The model under review builds one solid part; all positions refer to its coordinate system, in mm. A direction names the side the tool comes from. Round coordinates to 2 decimals unless told otherwise and drop trailing zeros. Loops run counter-clockwise (first coordinate to the right, second up) from the corner with the lowest first, then second, coordinate; pieces in that order, holes last. Notation, with made-up numbers: M 78.5,16 L 121.5,16 A30 cw 121.5,46 Z; hole C 55,12 d5. An arc over 180 degrees is marked long. Answer as a JSON object with one key per item and string values. Group by question number.
Item 1: To check wall thickness, follow line 1 (Y direction, x = -57, z = 9.5); line 2 (X direction, y = 184, z = 1); line 3 (X direction, y = 54, z = 6). State the ranges of each line that lie inside material, in increasing order.
Item 2: Consider section D-D (y = 131). Give the boundary of the cut face in (x, z), and give its area (3 significant figures).
Item 3: The part is to be moulded in two halves that separate along X. For faces 3 (the face through (60, 137, 8)), 4 (the face through (55, 135, 9)), 5 (the face through (-1, 92, 0)), 6 (the face through (-60, 135, 8)), say which applies: +X half, -X half, draft (parallel to the pull), parting line (faces both ways), or undercut.
Item 4: Tool access review of faces 1 (the face through (57.535, 153.585, 4.881)), 2 (the face through (-1, 92, 2)): name each direction out of +Z, -Z, +X, -X, +Y, -Y from which nothing blocks a thin tool from reaching the whole face with its end or side.
Item 5: Consider section A-A (y = 155.5). Give the boundary of the cut face in (x, z), and give its area (3 significant figures).
Item 6: Insertion check: P1, Ø6, axis at x = 16.5, y = 55.5, coming from the +Z side; P2, Ø5.5, axis at x = -56.5, z = 9.5, coming from the -Y side; P3, Ø1, axis at x = -49.5, z = 1.5, coming from the +Y side. Each pin has a flat end and moves straight along its axis. Give the tip position at first contact, or say it passes through.
Item 7: Consider section B-B (y = 192.5). Give the boundary of the cut face in (x, z).
Item 8: Consider section C-C (z = 9.5). Give the boundary of the cut face in (x, y).
Autodesk Inventor part; units mm, degrees
ref_plane "工作平面1" through (31, 232, 17) normal (1, 0, 0) x (0, 0, -1)
ref_plane "YZ Plane" through (0, 0, 0) normal (1, 0, 0) x (0, 1, 0)
ref_plane "XZ Plane" through (0, 0, 0) normal (0, 1, 0) x (-1, 0, 0)
sketch "草图1" plane through (0, 0, 0) normal (0, 0, 1) x (1, 0, 0)
  line L0 (-60, 0) -> (60, 0)
  line L1 (-60, 0) -> (-60, 232)
  line L2 (-60, 232) -> (60, 232)
  line L3 (60, 232) -> (60, 0)
  point P0 (0, 0)
  point P1 (0, 0)
  dimension "宽度" = 120
  dimension "长度" = 232
  dimension "d15" = 120
extrude "拉伸1" add sketch "草图1" along normal blind 2
sketch "草图2" plane through (0, 0, 2) normal (0, 0, 1) x (1, 0, 0)
  line L0 (-60, 0) -> (60, 0)
  line L1 (60, 0) -> (60, 232)
  line L2 (60, 232) -> (-60, 232)
  line L3 (-60, 232) -> (-60, 0)
  line L4 (-55, 232) -> (-55, 0)
  line L5 (0, 0) -> (0, 232) construction
  line L6 (55, 0) -> (55, 232)
  dimension "侧厚" = 5
extrude "拉伸2" add sketch "草图2" along normal blind 15 contours L3 L2 L4 L0 | L6 L2 L1 L0
sketch "草图3" plane through (60, 0, 0) normal (1, 0, 0) x (0, 0, -1)
  line L0 (0, 0) -> (0, 232)
  line L1 (0, 232) -> (-17, 232)
  line L2 (-17, 0) -> (-17, 232)
  line L3 (0, 0) -> (-17, 0)
  circle A0 centre (-9.5, 222) radius 5
  circle A1 centre (-9.5, 155.5) radius 5
  line L4 (-9.5, 222) -> (-9.5, 155.5) construction
  point P0 (0, 0)
  dimension "d16" = 10
  dimension "后孔位置" = 10
  dimension "上沿" = 7.5
  dimension "d29" = 10
  dimension "d30" = 66.5
extrude "拉伸3" cut sketch "草图3" against normal through all contours A0
sketch "草图4" plane through (0, 0, 2) normal (0, 0, 1) x (1, 0, 0)
  line L0 (-52, 232) -> (-52, 187)
  line L1 (-52, 187) -> (52, 187)
  line L2 (52, 187) -> (52, 232)
  line L3 (55, 232) -> (-55, 232)
  line L4 (0, 232) -> (0, 179.736464)
  line L5 (-52, 232) -> (52, 232)
  line L6 (55, 232) -> (55, 0)
  point P0 (0, 0)
  dimension "d26" = 45
  dimension "d39" = 3
extrude "拉伸4" cut sketch "草图4" along normal through all both and the other way through all
extrude "拉伸5" cut sketch "草图3" against normal through all contours A1
sketch "草图5" plane through (0, 0, 2) normal (0, 0, 1) x (1, 0, 0)
  line L0 (-55, 0) -> (-55, 232)
  line L1 (-52, 232) -> (-55, 232)
  line L2 (-45, 232) -> (-45, 92)
  line L3 (-25, 232) -> (-25, 92)
  line L4 (-45, 92) -> (-25, 92)
  point P0 (0, 0)
  dimension "d33" = 140
  dimension "d34" = 10
  dimension "d35" = 140
  dimension "d36" = 20
sketch "草图5 outline for 拉伸6" plane through (0, 0, 2) normal (0, 0, 1) x (1, 0, 0)
  line L0 (-45, 232) -> (-25, 232)
  line L1 (-25, 232) -> (-25, 92)
  line L2 (-25, 92) -> (-45, 92)
  line L3 (-45, 92) -> (-45, 232)
extrude "拉伸6" cut sketch "草图5 outline for 拉伸6" along normal through all both and the other way through all
sketch "草图6" plane through (0, 0, 2) normal (0, 0, 1) x (1, 0, 0)
  line L0 (60, 160.5) -> (60, 150.5)
  line L1 (55, 150.5) -> (55, 160.5)
  line L2 (55, 155.5) -> (0, 155.5) construction
  line L3 (0, 145.5) -> (0, 0) construction
  line L4 (55, 155.5) -> (55, 95.5) construction
  line L5 (55, 95.5) -> (0, 95.5) construction
  line L6 (-10, 95.5) -> (10, 95.5)
  line L7 (52, 187) -> (-25, 187)
  line L8 (10, 145.5) -> (10, 177) construction
  line L9 (0, 187) -> (0, 97)
  line L10 (0, 97) -> (20, 97)
  line L11 (20, 97) -> (20, 187)
  dimension "d40" = 60
  dimension "d46" = 90
  dimension "d47" = 20
  dimension "d48" = 10
extrude "拉伸7" cut sketch "草图6" against normal through all
sketch "草图7" plane through (0, 0, 2) normal (0, 0, 1) x (1, 0, 0)
  line L0 (60, 227) -> (60, 217)
  line L1 (55, 217) -> (55, 227)
  line L2 (-60, 232) -> (-60, 0)
  line L3 (60, 0) -> (60, 232)
  line L4 (-60, 0) -> (60, 0)
  line L5 (55, 222) -> (60, 222) construction
  circle A0 centre (0, 10) radius 2.5
  point P0 (0, 0)
  dimension "d49" = 5
  dimension "d50" = 212
extrude "拉伸8" cut sketch "草图7" against normal through all
sketch "草图8" plane through (0, 0, 2) normal (0, 0, 1) x (1, 0, 0)
  circle A0 centre (0, 10) radius 2.5
  line L0 (20, 187) -> (20, 97)
  line L1 (20, 97) -> (0, 97)
  line L2 (0, 97) -> (0, 187)
  line L3 (0, 187) -> (-25, 187)
  line L4 (-25, 187) -> (-25, 92)
  line L5 (-25, 92) -> (-45, 92)
  line L6 (-45, 92) -> (-45, 187)
  line L7 (-45, 187) -> (-52, 187)
  line L8 (-52, 187) -> (-52, 232)
  line L9 (-52, 232) -> (-55, 232)
  line L10 (-55, 232) -> (-55, 0)
  line L11 (-55, 0) -> (55, 0)
  line L12 (55, 0) -> (55, 232)
  line L13 (55, 232) -> (52, 232)
  line L14 (52, 232) -> (52, 187)
  line L15 (52, 187) -> (20, 187)
  line L16 (-60, 0) -> (-55, 0)
  line L17 (-55, 0) -> (-55, 232)
  line L18 (-55, 232) -> (-60, 232)
  line L19 (-60, 232) -> (-60, 0)
  line L20 (60, 0) -> (60, 232)
  line L21 (60, 232) -> (55, 232)
  line L22 (55, 232) -> (55, 0)
  line L23 (55, 0) -> (60, 0)
  line L24 (-15, 0) -> (-55, 40)
  line L25 (15, 0) -> (55, 40)
  line L26 (0, 0) -> (0, 39.183664) construction
  line L27 (-60, 232) -> (-60, 0)
  line L28 (-55, 40) -> (-60, 40)
  line L29 (-60, 40) -> (-60, 0)
  line L30 (-60, 0) -> (-15, 0)
  line L31 (15, 0) -> (60, 0)
  line L32 (55, 40) -> (60, 40)
  line L33 (60, 0) -> (60, 40)
  dimension "d53" = 30
  dimension "d55" = 40
extrude "拉伸9" cut sketch "草图8" along normal through all both and the other way through all contours L32 L20 L23 L12 | L12 L11 L25 | L11 L10 L24 | L16 L19 L28 L10
ref_plane "工作平面1" through (31, 232, 17) normal (1, 0, 0) x (0, 0, -1)
sketch "草图9" plane through (31, 232, 17) normal (1, 0, 0) x (0, 0, -1)
  line L0 (17, -192) -> (17, 0)
  line L1 (17, -56.209089) -> (-323, -175.94833)
  line L2 (-322.950917, -180.94833) -> (17, -61.209089)
  line L3 (17, -56.209089) -> (17, -61.209089)
  line L4 (-322.950917, -180.94833) -> (-323, -175.94833)
  point P0 (17, -232)
  dimension "d59" = 340
  dimension "d64" = 5
  dimension "d65" = 5
extrude "拉伸11" [suppressed]
properties part number "底板" material "木材(桦木)"
Geometry results:
{
 "1": {"line 1": "y = 40 to 150.5, 160.5 to 217, 227 to 232", "line 2": "x = -60 to -45, -25 to 0, 20 to 60", "line 3": "x = -60 to -55, 55 to 60"},
 "2": {"outline": "M -60,0 L -45,0 L -45,2 L -55,2 L -55,17 L -60,17 Z; M -25,0 L 0,0 L 0,2 L -25,2 Z; M 20,0 L 60,0 L 60,17 L 55,17 L 55,2 L 20,2 Z", "area": "310 mm^2"},
 "3": {"face 3": "+X half", "face 4": "undercut", "face 5": "draft", "face 6": "-X half"},
 "4": {"face 1": "+X, -X", "face 2": "+Z, +Y, -Y"},
 "5": {"outline": "M -60,0 L -45,0 L -45,2 L -55,2 L -55,4.5 L -60,4.5 Z; M -60,14.5 L -55,14.5 L -55,17 L -60,17 Z; M -25,0 L 0,0 L 0,2 L -25,2 Z; M 20,0 L 60,0 L 60,4.5 L 55,4.5 L 55,2 L 20,2 Z; M 55,14.5 L 60,14.5 L 60,17 L 55,17 Z", "area": "210 mm^2"},
 "6": {"P1": "stops at z = 2", "P2": "stops at y = 40", "P3": "stops at y = 187"},
 "7": {"outline": "M -60,0 L -52,0 L -52,2 L -55,2 L -55,17 L -60,17 Z; M 52,0 L 60,0 L 60,17 L 55,17 L 55,2 L 52,2 Z"},
 "8": {"outline": "M -60,40 L -55,40 L -55,150.5 L -60,150.5 Z; M -60,160.5 L -55,160.5 L -55,217 L -60,217 Z; M -60,227 L -55,227 L -55,232 L -60,232 Z; M 55,40 L 60,40 L 60,150.5 L 55,150.5 Z; M 55,160.5 L 60,160.5 L 60,217 L 55,217 Z; M 55,227 L 60,227 L 60,232 L 55,232 Z"}
}
